from build123d import *

# Parameters (mm, degrees)
SKETCH_R        = 2.425
PAD_DEPTH       = 10
SKETCH001_R     = 1.925
POCKET_DEPTH    = 12
SKETCH002_R     = 1.5
POCKET001_DEPTH = 12
SKETCH003_R     = 1.925
POCKET002_DEPTH = 12
SKETCH004_R     = 2.425
POCKET003_DEPTH = 12
SKETCH005_R     = 1.5
POCKET004_DEPTH = 12
POCKET005_DEPTH = 5
POCKET006_DEPTH = 12
POCKET007_DEPTH = 6


with BuildPart() as part:
    # Sketch → Pad (new body)
    with BuildSketch(Plane.XZ):
        with BuildLine():
            ThreePointArc((12, -31.811947), (33.448514, 6.098926), (0, 34))
            Line((0, 34), (-50.4621, 34))
            Line((-50.4621, 34), (-55.344463, 52.221225))
            Line((-55.344463, 52.221225), (-74.284202, 47.145798))
            Line((-74.284202, 47.145798), (-74.284202, 33.543798))
            Line((-74.284202, 33.543798), (-83, 24.828))
            Line((-83, 24.828), (-83, -54))
            Line((-83, -54), (12, -54))
            Line((12, -54), (12, -31.811947))
        make_face()
        Circle(SKETCH_R, mode=Mode.SUBTRACT)
    extrude(amount=PAD_DEPTH)

    # Sketch001 (on Face12 of Pad) → Pocket (cut)
    with BuildSketch(Plane.XZ.offset(10)):
        with Locations((-69, -49)):
            Circle(SKETCH001_R)
        with Locations((-23, -49)):
            Circle(SKETCH001_R)
        with Locations((2, -49)):
            Circle(SKETCH001_R)
    extrude(amount=-POCKET_DEPTH, mode=Mode.SUBTRACT)

    # Sketch002 (on Face5 of Pocket) → Pocket001 (cut)
    with BuildSketch(Plane.XZ.offset(10)):
        with Locations((-43, -1)):
            Circle(SKETCH002_R)
        with BuildLine():
            ThreePointArc((-62, -3.8), (-73.2, -15), (-62, -26.2))
            Line((-62, -26.2), (-52, -26.2))
            ThreePointArc((-52, -26.2), (-40.8, -15), (-52, -3.8))
            Line((-52, -3.8), (-62, -3.8))
        make_face()
        with BuildLine():
            ThreePointArc((-77.5, -29), (-79, -30.5), (-77.5, -32))
            Line((-77.5, -32), (-67.5, -32))
            ThreePointArc((-67.5, -32), (-66, -30.5), (-67.5, -29))
            Line((-67.5, -29), (-77.5, -29))
        make_face()
        with BuildLine():
            ThreePointArc((-46.5, -29), (-48, -30.5), (-46.5, -32))
            Line((-46.5, -32), (-36.5, -32))
            ThreePointArc((-36.5, -32), (-35, -30.5), (-36.5, -29))
            Line((-36.5, -29), (-46.5, -29))
        make_face()
        with BuildLine():
            ThreePointArc((-77.5, 2), (-79, 0.5), (-77.5, -1))
            Line((-77.5, -1), (-67.5, -1))
            ThreePointArc((-67.5, -1), (-66, 0.5), (-67.5, 2))
            Line((-67.5, 2), (-77.5, 2))
        make_face()
    extrude(amount=-POCKET001_DEPTH, mode=Mode.SUBTRACT)

    # Sketch003 (on Face5 of Pocket001) → Pocket002 (cut)
    with BuildSketch(Plane.XZ.offset(10)):
        with Locations((-67, 11)):
            Circle(SKETCH003_R)
    extrude(amount=-POCKET002_DEPTH, mode=Mode.SUBTRACT)

    # Sketch004 (on Face5 of Pocket002) → Pocket003 (cut)
    with BuildSketch(Plane.XZ.offset(10)):
        with Locations((-30.641778, 25.711504)):
            Circle(SKETCH004_R)
    extrude(amount=-POCKET003_DEPTH, mode=Mode.SUBTRACT)

    # Sketch005 (on Face5 of Pocket003) → Pocket004 (cut)
    with BuildSketch(Plane.XZ.offset(10)):
        with Locations((-57.838829, 47.234623)):
            Circle(SKETCH005_R)
        with Locations((-52.921267, 28.882032)):
            Circle(SKETCH005_R)
        with Locations((-71.317, 26.8)):
            Circle(SKETCH005_R)
    extrude(amount=-POCKET004_DEPTH, mode=Mode.SUBTRACT)

    # Sketch006 (on Face5 of Pocket004) → Pocket005 (cut)
    with BuildSketch(Plane.XZ.offset(10)):
        Polygon((-54.82737, 46.427705), (-55.634288, 49.439164), (-58.645747, 50.246082), (-60.850288, 48.041541), (-60.04337, 45.030082), (-57.031911, 44.223164), align=None)
        Polygon((-50.716726, 31.086573), (-53.728185, 31.893491), (-55.932726, 29.68895), (-55.125808, 26.677491), (-52.114349, 25.870573), (-49.909808, 28.075114), align=None)
        Polygon((-73.521541, 24.595459), (-70.510082, 23.788541), (-68.305541, 25.993082), (-69.112459, 29.004541), (-72.123918, 29.811459), (-74.328459, 27.606918), align=None)
    extrude(amount=-POCKET005_DEPTH, mode=Mode.SUBTRACT)

    # Sketch007 (on Face5 of Pocket005) → Pocket006 (cut)
    with BuildSketch(Plane.XZ.offset(10)):
        with BuildLine():
            ThreePointArc((-76, 23), (-78, 25), (-80, 23))
            Line((-80, 23), (-80, 11))
            ThreePointArc((-80, 11), (-78, 9), (-76, 11))
            Line((-76, 11), (-76, 23))
        make_face()
    extrude(amount=-POCKET006_DEPTH, mode=Mode.SUBTRACT)

    # Sketch008 (on Face4 of Pocket006) → Pocket007 (cut)
    with BuildSketch(Plane(origin=(0, 0, 0), x_dir=(1, 0, 0), z_dir=(0, 1, 0))):
        Polygon((-40.3, -0.558846), (-40.3, 2.558846), (-43, 4.117691), (-45.7, 2.558846), (-45.7, -0.558846), (-43, -2.117691), align=None)
    extrude(amount=-POCKET007_DEPTH, mode=Mode.SUBTRACT)


solid = part.part
The model under review builds one solid part; all positions refer to its coordinate system, in mm. A direction names the side the tool comes from. Give positions to 0.01 mm unless a question says otherwise; leave off trailing zeros. Order: outer loops, then holes, each group sorted by start corner. A loop starts at its lowest first (then second) coordinate and runs counter-clockwise, first axis right, second up. Notation, with made-up numbers: M 19,20 L 61,20 A15 cw 61,44 Z; hole C -10.5,39 d11. An arc over 180 degrees is marked long. Answer in a Markdown table with one row per item. Add a question column.
1. Add section D-D on z = 38. State the section outline as (x, y) points, plus the area to 3 significant figures.
2. Machinability: for faces 1 (the flat face through (-25, -10, -12)), 2 (the cylindrical face through (-78, -5, 25)), 3 (the flat face through (-52.201, -7.535, 31.484)), which of the approach directions +Z, -Z, +X, -X, +Y, -Y give a long, thin tool a straight path to every point of the face, cutting with its end or side? Answer none if there is none.
3. For pin 1 Ø4.5 at (x, z) = (2, -49) entering from +Y; pin 2 Ø3 at (y, z) = (-4.5, 17) entering from +X; pin 3 Ø5 at (y, z) = (-5, 38) entering from -X; pin 4 Ø4 at (x, y) = (10, -6.5) entering from +Z, all flat-tipped, find the tip position at first contact; note any pin that passes through.
4. Mouldability with a two-part tool opening along X and no side actions: class faces 4 (the flat face through (-59, -5, 49)), 5 (the flat face through (-36, -5, -54)), 6 (the cylindrical face through (33.56, -4.93, 5.45)) as released by +X, released by -X, zero draft, split by the parting line, or undercut.
5. Add section C-C on x = -8.5. State the section outline as (y, z) points, plus the area to 3 significant figures.
6. Add section B-B on z = -11.5. State the section outline as (x, y) points, plus the area to 3 significant figures.
7. To check wall thickness, follow line 1 along Z through (x, y) = (-69, -4.25) (3 decimals); line 2 along X through (y, z) = (-9.25, 12); line 3 along Z through (x, y) = (-37.5, -0.25). State the ranges of each line that lie inside material, in increasing order.
8. Add section A-A on x = -23. State the section outline as (y, z) points (3 decimals).
The answers:
| question | item | result |
|---|---|---|
| 1 | outline | M -74.28,-10 L -51.53,-10 L -51.53,0 L -74.28,0 Z |
| 1 | area | 228 mm2 |
| 2 | face 1 | +Z, -Z, +X, -X, -Y |
| 2 | face 2 | +Y, -Y |
| 2 | face 3 | -Y |
| 3 | pin 1 | y = 0 |
| 3 | pin 2 | x = 30.26 |
| 3 | pin 3 | x = -74.28 |
| 3 | pin 4 | z = 33.05 |
| 4 | face 4 | undercut |
| 4 | face 5 | zero draft |
| 4 | face 6 | released by +X |
| 5 | outline | M -10,-54 L 0,-54 L 0,34 L -10,34 Z |
| 5 | area | 880 mm2 |
| 6 | outline | M -83,-10 L -72.64,-10 L -72.64,0 L -83,0 Z; M -41.36,-10 L 32,-10 L 32,0 L -41.36,0 Z |
| 6 | area | 837 mm2 |
| 7 | line 1 | -54 to -50.925, -47.075 to -32, -29 to -23.743, -6.257 to -1, 2 to 48.562 |
| 7 | line 2 | -83 to -80, -76 to -68.64, -65.36 to 31.81 |
| 7 | line 3 | -54 to -32, -29 to 34 |
| 8 | outline | M -10,-54 L 0,-54 L 0,-50.925 L -10,-50.925 Z; M -10,-47.075 L 0,-47.075 L 0,34 L -10,34 Z |
